Model file for the job. Use its own axes, mm. Face numbers are marked on the shaded views. Round coordinates to 2 decimals unless told otherwise and drop trailing zeros. Write each loop counter-clockwise with the first axis right and the second up, starting at its lowest first coordinate (ties: lowest second). Pieces come first, ordered by that corner, then holes. Notation, with made-up numbers: (-11.5, 72.5) - (33.5, 72.5) arc R26 cw to (33.5, 87.5) - close; hole circle Ø8 at (-37.75, 16). An arc over 180 degrees is marked (long way). One line per item, written item: value.
from build123d import *

# Parameters (mm, degrees)
EXTRUIR1_DEPTH      = 16
EXTRUIR2_REACH      = 58.273
EXTRUIR2_END_RADIUS = 19
EXTRUIR2_START      = 25
CROQUIS2_R          = 4
REDONDEO1_R         = 3
REDONDEO2_R         = 0.5
EXTRUIR3_START      = -16
EXTRUIR3_DEPTH      = 16


with BuildPart() as part:
    # Croquis1 → Extruir1 (new body)
    with BuildSketch(Plane(origin=(0, 0, 0), x_dir=(1, 0, 0), z_dir=(0, 1, 0))):
        with BuildLine():
            Line((16.454482672, 9.5), (13.856406461, 8))
            ThreePointArc((13.856406461, 8), (0, -16), (-13.856406461, 8))
            Line((-13.856406461, 8), (-16.454482672, 9.5))
            ThreePointArc((-16.454482672, 9.5), (0, -19), (16.454482672, 9.5))
        make_face()
    extrude(amount=EXTRUIR1_DEPTH)

    # Extruir2: up to this cylinder (the profile starts outside it)
    extruir2_end = Plane(origin=(0, 8, 0), z_dir=(0, -1, 0)) * Cylinder(EXTRUIR2_END_RADIUS, 155.546, mode=Mode.PRIVATE)
    # Croquis2 → Extruir2 (add, up to the surface)
    with BuildSketch(Plane.XY.offset(EXTRUIR2_START), mode=Mode.PRIVATE) as extruir2_sk1:
        with Locations((0, 8)):
            Circle(CROQUIS2_R)
    extruir2_tool1 = extrude(extruir2_sk1.sketch, amount=-EXTRUIR2_REACH, mode=Mode.PRIVATE) - extruir2_end
    add(extruir2_tool1.solids().sort_by_distance((0, 8, 25))[0])

    # Redondeo1
    redondeo1_edges = [part.edges().sort_by_distance(p)[0] for p in [
        (13.856406461, 8, -8),
        (-13.856406461, 8, -8),
    ]]
    fillet(redondeo1_edges, radius=REDONDEO1_R)

    # Redondeo2
    redondeo2_edges = [part.edges().sort_by_distance(p)[0] for p in [
        (16.454482672, 8, -9.5),
        (-16.454482672, 8, -9.5),
    ]]
    fillet(redondeo2_edges, radius=REDONDEO2_R)

    # Croquis3 → Extruir3 (add)
    with BuildSketch(Plane(origin=(0, 16, 0), x_dir=(1, 0, 0), z_dir=(0, 1, 0)).offset(EXTRUIR3_START)):
        with BuildLine():
            Line((-18.548840002, -4.115888068), (-14, -24.615888068))
            Line((-14, -24.615888068), (14, -24.615888068))
            Line((14, -24.615888068), (18.548840002, -4.115888068))
            Line((18.548840002, -4.115888068), (15.461547963, -4.115888068))
            ThreePointArc((15.461547963, -4.115888068), (0, -16), (-15.461547963, -4.115888068))
            Line((-15.461547963, -4.115888068), (-18.548840002, -4.115888068))
        make_face()
    extrude(amount=EXTRUIR3_DEPTH)


solid = part.part
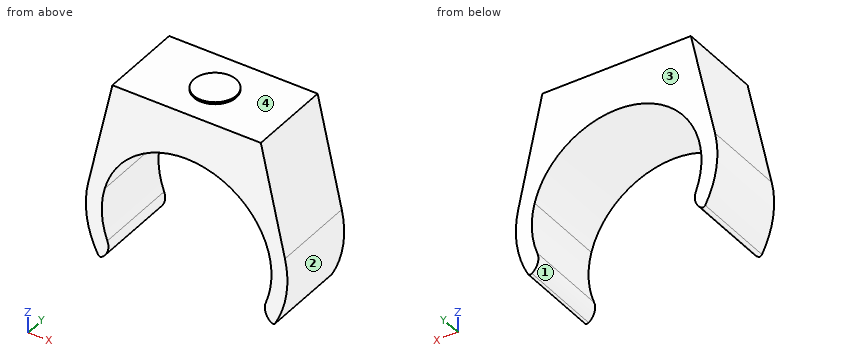
1. Drop flat-ended pins along their axis: pin 1 (5 mm diameter, centred on y = 2.5, z = 19.5, fed in from -X); pin 2 (10 mm diameter, centred on x = -8.5, z = -1.5, fed in from +Y); pin 3 (3 mm diameter, centred on x = 8, y = 8, fed in from -Z); pin 4 (5 mm diameter, centred on x = -12.5, y = 7.5, fed in from -Z). Give the stop position or say it passes through.
Report:
pin 1: x = -15.69
pin 2: through
pin 3: z = 12.87
pin 4: z = -7.99
2. Band-saw the part on D-D on z = 22. Write the cut outline in (x, y).
Report:
outline: (-14.58, 0) - (14.58, 0) - (14.58, 16) - (-14.58, 16) - close
3. Mould opens along Z. For the marked faces 1, 2, 3 and 4 say: released by +Z, released by -Z, zero draft, split by the parting line, or undercut.
Report:
face 1: undercut
face 2: split by the parting line
face 3: zero draft
face 4: released by +Z
4. Band-saw the part on C-C on z = 7. Write the cut outline in (x, y).
Report:
outline: (-17.91, 0) - (-14.39, 0) - (-14.39, 16) - (-17.91, 16) - close; (14.39, 0) - (17.91, 0) - (17.91, 16) - (14.39, 16) - close
5. Band-saw the part on B-B on x = 0. Write the cut outline in (y, z).
Report:
outline: (0, 16) - (16, 16) - (16, 24.62) - (12, 24.62) - (12, 25) - (4, 25) - (4, 24.62) - (0, 24.62) - close
6. Wall check: probe 1 along X at (y, z) = (14.75, 10.5); probe 2 along X at (y, z) = (8.75, -7); probe 3 along Z at (x, y) = (1, 6.5). Give the ranges that are in metal, low to high. Write a range as [from, to].
Report:
probe 1: [-17.13, -12.07], [12.07, 17.13]
probe 2: [-17.66, -14.76], [14.76, 17.66]
probe 3: [15.97, 25]
7. Band-saw the part on A-A on z = 10.5. Write the cut outline in (x, y).
Report:
outline: (-17.13, 0) - (-12.07, 0) - (-12.07, 16) - (-17.13, 16) - close; (12.07, 0) - (17.13, 0) - (17.13, 16) - (12.07, 16) - close
